Model file for the job. Use its own axes, mm. Face numbers are marked on the shaded views. Coordinates: 2 decimals unless noted, no trailing zeros. Loops run counter-clockwise (first coordinate to the right, second up) from the corner with the lowest first, then second, coordinate; pieces in that order, holes last. Notation, with made-up numbers: M 49.5,64 L 57.5,64 A17 cw 57.5,85 Z; hole C -0.5,82 d5. An arc over 180 degrees is marked long. Write item = value, one per line. Start each with the question number.
from build123d import *

# Parameters (mm, degrees)
SKETCH1_W           = 144.78
SKETCH1_H           = 50.8
BOSS_EXTRUDE1_DEPTH = 3.81
SKETCH2_W           = 3.81
SKETCH2_H           = 12.7
BOSS_EXTRUDE2_DEPTH = 17.78
CUT_EXTRUDE1_REACH  = 146.78
SKETCH4_W           = 10.668
SKETCH4_H           = 20.32
CUT_EXTRUDE2_DEPTH  = 22.59
FILLET3_R           = 5.08
FILLET4_R           = 2.54


with BuildPart() as part:
    # Sketch1 → Boss-Extrude1 (new body)
    with BuildSketch(Plane(origin=(0, 0, 0), x_dir=(1, 0, 0), z_dir=(0, 1, 0))):
        Rectangle(SKETCH1_W, SKETCH1_H)
    extrude(amount=BOSS_EXTRUDE1_DEPTH)

    # Sketch2 → Boss-Extrude2 (add)
    with BuildSketch(Plane(origin=(0, 3.81, 0), x_dir=(1, 0, 0), z_dir=(0, 1, 0))):
        with Locations((70.485, 0)):
            Rectangle(SKETCH2_W, SKETCH2_H)
    extrude(amount=BOSS_EXTRUDE2_DEPTH)

    # Sketch3 → Cut-Extrude1 (cut, up to next)
    with BuildSketch(Plane(origin=(72.39, 0, 0), x_dir=(0, 0, -1), z_dir=(1, 0, 0)), mode=Mode.PRIVATE) as cut_extrude1_sk1:
        with BuildLine():
            Line((-2.54, 21.59), (2.54, 21.59))
            Line((2.54, 21.59), (2.54, 19.05))
            ThreePointArc((2.54, 19.05), (0, 16.51), (-2.54, 19.05))
            Line((-2.54, 19.05), (-2.54, 21.59))
        make_face()
    cut_extrude1_tool1 = extrude(cut_extrude1_sk1.sketch, amount=-CUT_EXTRUDE1_REACH, mode=Mode.PRIVATE) & part.part
    add(cut_extrude1_tool1.solids().sort_by_distance((72.39, 19.287109, 0))[0], mode=Mode.SUBTRACT)

    # Sketch4 → Cut-Extrude2 (cut, through all)
    with BuildSketch(Plane.XZ):
        with Locations((-46.976, 0)):
            Rectangle(SKETCH4_W, SKETCH4_H)
    extrude(amount=-CUT_EXTRUDE2_DEPTH, mode=Mode.SUBTRACT)

    # Fillet3
    fillet3_edges = [part.edges().sort_by_distance(p)[0] for p in [
        (72.39, 1.905, 25.4),
        (-72.39, 1.905, 25.4),
        (-72.39, 1.905, -25.4),
        (72.39, 1.905, -25.4),
    ]]
    fillet(fillet3_edges, radius=FILLET3_R)

    # Fillet4
    fillet4_edges = [part.edges().sort_by_distance(p)[0] for p in [
        (-52.31, 0, 0),
        (-46.976, 0, -10.16),
        (-41.642, 0, 0),
        (-46.976, 0, 10.16),
        (-72.39, 0, 0),
        (72.39, 0, 0),
        (0, 0, 25.4),
        (0, 0, -25.4),
        (70.902102448, 0, -23.912102448),
        (70.902102448, 0, 23.912102448),
        (-70.902102448, 0, 23.912102448),
        (-70.902102448, 0, -23.912102448),
    ]]
    fillet(fillet4_edges, radius=FILLET4_R)


solid = part.part
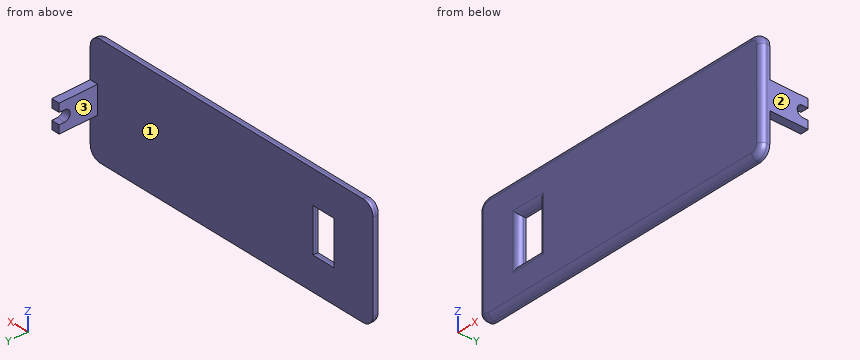
Item 1: Probe L1, parallel to X at y = 3.25, z = 5.5; L2, parallel to Y at x = -49, z = -20; L3, parallel to X at y = 4.25, z = -1. List the from-to ranges inside material, lowest first.
Item 2: Cut at C-C (z = -16). Give the cut face in (x, y), plus the area to 3 significant figures.
Item 3: Cut at A-A (z = 0). Give the cut face in (x, y), plus the area to 3 significant figures.
Item 4: Pull direction X, two halves, no side cores. Call the marked faces 1, 2 and 3: +X half, -X half, draft (parallel to the pull), parting line (faces both ways), or undercut.
Item 5: Cut at B-B (x = 25). Give the cut face in (y, z).
Item 6: Cut at D-D (y = 8.75). Give the cut face in (x, z), plus the area to 3 significant figures.
Item 7: Pin check, flat tips, straight feed: pin 1 Ø1.1 at (x, y) = (70, 16.5) entering from +Z; pin 2 Ø2 at (x, z) = (-42, -4) entering from +Y; pin 3 Ø3 at (x, y) = (71.5, 20.5) entering from -Z. Stop position of each tip, or through.
Reported:
q1.L1 = -72.39 to -52.31, -41.64 to 72.39
q1.L2 = 0 to 3.81
q1.L3 = 68.58 to 72.39
q2.outline = M -72.39,2.54 A2.54 ccw -69.85,0 L 69.85,0 A2.54 ccw 72.39,2.54 L 72.39,3.81 L -72.39,3.81 Z
q2.area = 549 mm^2
q3.outline = M -72.39,2.54 A2.54 ccw -69.85,0 L -54.85,0 A2.54 ccw -52.31,2.54 L -52.31,3.81 L -72.39,3.81 Z; M -41.64,2.54 A2.54 ccw -39.1,0 L 69.85,0 A2.54 ccw 72.39,2.54 L 72.39,16.51 L 68.58,16.51 L 68.58,3.81 L -41.64,3.81 Z
q3.area = 554 mm^2
q4.face_1 = draft
q4.face_2 = +X half
q4.face_3 = -X half
q5.outline = M 0,-22.86 A2.54 ccw 2.54,-25.4 L 3.81,-25.4 L 3.81,25.4 L 2.54,25.4 A2.54 ccw 0,22.86 Z
q6.outline = M 68.58,-6.35 L 72.39,-6.35 L 72.39,6.35 L 68.58,6.35 Z
q6.area = 48.4 mm^2
q7.pin_1 = 6.35
q7.pin_2 = 3.81
q7.pin_3 = -6.35
